Design review of the part built by this model. Coordinates are the model's own, in mm. A direction names the side the tool comes from. Round coordinates to 2 decimals unless told otherwise and drop trailing zeros. Order: outer loops, then holes, each group sorted by start corner. A loop starts at its lowest first (then second) coordinate and runs counter-clockwise, first axis right, second up. Notation, with made-up numbers: (-26, -36) - (6, -36) arc R17 ccw to (6, -21) - close; hole circle Ø5 at (-5.75, 70.25). An arc over 180 degrees is marked (long way). Answer as a JSON object with one key per item and string values. Group by question number.
from build123d import *

# Parameters (mm, degrees)
BOSS_EXTRUDE1_DEPTH      = 14
SKETCH3_R                = 4.125
CUT_EXTRUDE1_DEPTH       = 6
SKETCH5_R                = 1.125
CUT_EXTRUDE2_DEPTH       = 15
FILLET1_R                = 1
BOSS_EXTRUDE3_DEPTH      = 20
BOSS_EXTRUDE3_DEPTH_BACK = 34
SKETCH7_W                = 46.707438453
SKETCH7_H                = 20
CUT_EXTRUDE3_DEPTH       = 30
BOSS_EXTRUDE4_DEPTH      = 3
BOSS_EXTRUDE5_START      = -54
BOSS_EXTRUDE5_DEPTH      = 3
CUT_EXTRUDE5_REACH       = 111.564
SKETCH15_W               = 26.880557743
SKETCH15_H               = 40.856784115
CUT_EXTRUDE6_REACH       = 113.249
SKETCH16_R               = 1.6
CUT_EXTRUDE7_DEPTH       = 112.248863996
CUT_EXTRUDE8_DEPTH       = 106.753443393
SKETCH20_R               = 2.6
CUT_EXTRUDE9_DEPTH       = 106.753443393


with BuildPart() as part:
    # Sketch1 → Boss-Extrude1 (new body)
    with BuildSketch(Plane(origin=(0, 0, 0), x_dir=(1, 0, 0), z_dir=(0, 1, 0))):
        with BuildLine():
            Line((47.5, -78.442713945), (47.5, -38.442713945))
            ThreePointArc((47.5, -38.442713945), (23.122023742, 0), (47.5, 38.442713945))
            Line((47.5, 38.442713945), (47.5, 50))
            Line((47.5, 50), (42.5, 50))
            Line((42.5, 50), (0, 0))
            Line((0, 0), (35.1, -73.422380253))
            Line((35.1, -73.422380253), (35.1, -93.442713945))
            Line((35.1, -93.442713945), (37.5, -93.442713945))
            Line((37.5, -93.442713945), (47.5, -93.442713945))
            Line((47.5, -93.442713945), (47.5, -78.442713945))
        make_face()
    extrude(amount=BOSS_EXTRUDE1_DEPTH)

    # Sketch3 → Cut-Extrude1 (cut)
    with BuildSketch(Plane.XZ):
        with BuildLine():
            Line((33.254958794, 84.403112572), (36.18509612, 92.428977457))
            Line((36.18509612, 92.428977457), (44.88509612, 92.428977457))
            Line((44.88509612, 92.428977457), (46.13509612, 88.028977457))
            Line((46.13509612, 88.028977457), (46.13509612, 70.028977457))
            Line((46.13509612, 70.028977457), (44.820911197, 53.062159312))
            ThreePointArc((44.820911197, 53.062159312), (40.059955227, 48.679043991), (35.34566343, 53.112310791))
            Line((35.34566343, 53.112310791), (33.254958794, 84.403112572))
        make_face()
        with Locations(Location((40.08509612, 83.428977457, 0), (0, 0, 90))):
            Circle(SKETCH3_R, mode=Mode.SUBTRACT)
    extrude(amount=-CUT_EXTRUDE1_DEPTH, mode=Mode.SUBTRACT)

    # Sketch5 → Cut-Extrude2 (cut)
    with BuildSketch(Plane.XZ.offset(-6)):
        with Locations(Location((40.08509612, 63.428977457, 0), (0, 0, 270))):
            Circle(SKETCH5_R)
        with Locations(Location((40.08509612, 58.928977457, 0), (0, 0, 270))):
            Circle(SKETCH5_R)
        with Locations(Location((40.08509612, 53.428977457, 0), (0, 0, 270))):
            Circle(SKETCH5_R)
    extrude(amount=-CUT_EXTRUDE2_DEPTH, mode=Mode.SUBTRACT)

    # Fillet1
    fillet1_edges = [part.edges().sort_by_distance(p)[0] for p in [
        (21.25, 0, -25),
        (45, 0, -50),
        (47.5, 0, -44.221356973),
        (23.122023742, 14, 0),
        (23.122023742, 0, 0),
        (47.5, 0, 65.942713945),
        (47.5, 14, -44.221356973),
        (42.5, 7, -50),
        (47.5, 7, -50),
        (47.5, 7, -38.442713945),
        (47.5, 7, 38.442713945),
        (45, 14, -50),
        (21.25, 14, -25),
        (47.5, 14, 65.942713945),
    ]]
    fillet(fillet1_edges, radius=FILLET1_R)

    # Sketch6 → Boss-Extrude3 (add, two sides: drawn at the far end of the back side and taken through both)
    with BuildSketch(Plane.XZ.offset(-BOSS_EXTRUDE3_DEPTH_BACK)):
        with BuildLine():
            Line((-40.458581161, -20.077158004), (-49.887563088, -23.407968691))
            Line((-49.887563088, -23.407968691), (34.124921356, 71.382705183))
            Line((34.124921356, 71.382705183), (0, 0))
            ThreePointArc((0, 0), (-10.212270894, 1.77453397), (-20.560220827, 2.374016932))
            Line((-20.560220827, 2.374016932), (-40.458581161, -20.077158004))
        make_face()
    extrude(amount=BOSS_EXTRUDE3_DEPTH + BOSS_EXTRUDE3_DEPTH_BACK)

    # Sketch7 → Cut-Extrude3 (cut)
    with BuildSketch(Plane(origin=(-16.32086192, 0, 14.465095586), x_dir=(0.6632786778078259, 0, 0.7483724978682089), z_dir=(-0.7483724978682089, 0, 0.6632786778078259))):
        with Locations((52.701466874, 24)):
            Rectangle(SKETCH7_W, SKETCH7_H)
        with Locations((52.701466874, -10)):
            Rectangle(SKETCH7_W, SKETCH7_H)
    extrude(amount=-CUT_EXTRUDE3_DEPTH, mode=Mode.SUBTRACT)

    # Sketch10 → Boss-Extrude4 (add)
    with BuildSketch(Plane.XZ.offset(20)):
        Polygon((-49.887563088, -23.407968691), (-42.403838109, -30.040755469), (0, 0), (-16.723629197, 14.010656202), align=None)
    extrude(amount=-BOSS_EXTRUDE4_DEPTH)

    # Sketch10<2> → Boss-Extrude5 (add)
    with BuildSketch(Plane.XZ.offset(20).offset(BOSS_EXTRUDE5_START)):
        Polygon((-49.887563088, -23.407968691), (-42.403838109, -30.040755469), (0, 0), (-16.723629197, 14.010656202), align=None)
    extrude(amount=BOSS_EXTRUDE5_DEPTH)

    # Cut-Extrude5: up to this face of the body (flat: up to its plane)
    cut_extrude5_end = Plane(part.part.faces().sort_by_distance((40.08509612, 0, 83.428977457))[0])
    # Sketch15 → Cut-Extrude5 (cut, up to the picked face)
    with BuildSketch(Plane(origin=(0, 6, 0), x_dir=(-1, 0, 0), z_dir=(0, -1, 0)), mode=Mode.PRIVATE) as cut_extrude5_sk1:
        with Locations((-44.420319758, -91.811097241)):
            Rectangle(SKETCH15_W, SKETCH15_H)
    cut_extrude5_tool1 = split(extrude(cut_extrude5_sk1.sketch, amount=CUT_EXTRUDE5_REACH, mode=Mode.PRIVATE), bisect_by=cut_extrude5_end, keep=Keep.BOTH, mode=Mode.PRIVATE)
    add(cut_extrude5_tool1.solids().sort_by(Axis((44.42032, 6, 91.811097), (0, -1, 0)))[0], mode=Mode.SUBTRACT)

    # Sketch16 → Cut-Extrude6 (cut, up to next)
    with BuildSketch(Plane(origin=(0, 14, 0), x_dir=(1, 0, 0), z_dir=(0, 1, 0)), mode=Mode.PRIVATE) as cut_extrude6_sk1:
        with Locations(Location((40.08509612, -83.428977457, 0), (0, 0, 270))):
            Circle(SKETCH16_R)
    cut_extrude6_tool1 = extrude(cut_extrude6_sk1.sketch, amount=-CUT_EXTRUDE6_REACH, mode=Mode.PRIVATE) & part.part
    add(cut_extrude6_tool1.solids().sort_by_distance((40.085096, 14, 83.428977))[0], mode=Mode.SUBTRACT)

    # Sketch18 → Cut-Extrude7 (cut, through all)
    with BuildSketch(Plane(origin=(0, 0, 0), x_dir=(-0.4313049702307203, 0, -0.902206197415135), z_dir=(0.902206197415135, 0, -0.4313049702307203))):
        Polygon((-39.631978176, 14), (0, 14), (0, 0), (-37.370332893, 0), (-34.306310934, -43.962437664), (76.533165387, -56.066116366), (76.533165387, 47.196171587), (-42.014855984, 38.664050635), align=None)
    extrude(amount=-CUT_EXTRUDE7_DEPTH, mode=Mode.SUBTRACT)

    # Sketch19 → Cut-Extrude8 (cut, through all)
    with BuildSketch(Plane(origin=(0, 0, 0), x_dir=(-1, 0, 0), z_dir=(0, -1, 0))):
        Polygon((16.32086192, -14.465095586), (0, 0), (18.115156321, 31.62995048), (35.203757787, 6.840338193), align=None)
    extrude(amount=-CUT_EXTRUDE8_DEPTH, mode=Mode.SUBTRACT)

    # Sketch20 → Cut-Extrude9 (cut, through all)
    with BuildSketch(Plane(origin=(0, 0, 0), x_dir=(-1, 0, 0), z_dir=(0, -1, 0))):
        with Locations(Location((5.733478103, -15.103299236, 0), (0, 0, 90))):
            Circle(SKETCH20_R)
        with Locations(Location((-4.215702064, -26.328886704, 0), (0, 0, 90))):
            Circle(SKETCH20_R)
    extrude(amount=-CUT_EXTRUDE9_DEPTH, mode=Mode.SUBTRACT)


solid = part.part
1. Tool access review of faces 1 (the flat face through (21.396, 6.916, -25.171)), 2 (the flat face through (35.1, 10, 83)), 3 (the flat face through (34.744, 2.958, 62.12)): name each direction out of +Z, -Z, +X, -X, +Y, -Y from which nothing blocks a thin tool from reaching the whole face with its end or side.
2. Take a section at A-A, the plane y = 9.25. Count the separate pieces of the cut face and the enclosed holes in it, then the cut area to 3 significant figures.
3. Take a section at B-B, the plane y = 2.5. Give the boundary of the cut face in (x, z), then the cut area to 3 significant figures.
4. Mouldability with a two-part tool opening along Z and no side actions: class faces 4 (the flat face through (41, 6, 71)), 5 (the flat face through (41, 10, 93.443)), 6 (the cylindrical face through (-6.73, 6.9, 12.7)), 7 (the cylindrical face through (20.887, 13.715, -24.109)) as pulls with the +Z half, pulls with the -Z half, needs draft (parallel to the pull), parting line crosses it, or undercut.
5. Clearance check with flat-ended pins moving along their axes: P1, Ø4, axis at y = 10, z = 85.5, coming from the -X side; P2, Ø5, axis at x = 32, y = 11, coming from the -Z side; P3, Ø8, axis at y = 7, z = 37, coming from the -X side. State where each tip first meets the part, or that it passes through.
6. To check wall thickness, follow line 1 (Z direction, x = 39.5, y = 10.25); line 2 (X direction, y = 8.5, z = 79); line 3 (X direction, y = 8.5, z = 59). State the ranges of each line that lie inside material, in increasing order. Write a range as from..to.
7. Take a section at C-C, the plane z = 46. Give the boundary of the cut face in (x, y).
Response values:
{
 "1": {"face 1": "-Z, -X, +Y, -Y", "face 2": "+Z, -X, +Y, -Y", "face 3": "+Z, -Y"},
 "2": {"separate pieces": "1", "enclosed holes": "6", "area": "3,180 mm2"},
 "3": {"outline": "(-16.32, 14.47) - (0, 0) - (42.2, -49.65) arc R1 ccw to (42.96, -50) - (46.5, -50) arc R1 ccw to (47.5, -49) - (47.5, -39.07) arc R1 ccw to (46.94, -38.17) arc R42.5 cw to (46.94, 38.17) arc R1 ccw to (47.5, 39.07) - (47.5, 71.38) - (46.14, 71.38) - (46.14, 70.03) - (44.82, 53.06) arc R4.75 cw to (35.35, 53.11) - (34.12, 71.38) - close; hole circle Ø5.2 at (-5.73, 15.1); hole circle Ø5.2 at (4.22, 26.33)", "area": "2,700 mm2"},
 "4": {"face 4": "needs draft", "face 5": "pulls with the +Z half", "face 6": "undercut", "face 7": "pulls with the -Z half"},
 "5": {"P1": "x = 35.1", "P2": "z = -40.59", "P3": "x = 0.11"},
 "6": {"line 1": "-46.47..-33.52, 33.52..52.47, 54.39..57.97, 59.89..62.47, 64.39..81.94, 84.92..93.44", "line 2": "35.1..47.5", "line 3": "23.15..38.96, 41.21..47.5"},
 "7": {"outline": "(11.63, 0) - (46.5, 0) arc R1 ccw to (47.5, 1) - (47.5, 13) arc R1 ccw to (46.5, 14) - (11.63, 14) - close"}
}
